Read the model definition and answer for the solid it produces. Units are mm, in the model's axes. Face numbers are marked on the shaded views. A direction names the side the tool comes from. Give positions to 0.01 mm unless a question says otherwise; leave off trailing zeros. Write each loop counter-clockwise with the first axis right and the second up, starting at its lowest first coordinate (ties: lowest second). Pieces come first, ordered by that corner, then holes. Notation, with made-up numbers: M 24.25,8.5 L 49.25,8.5 A18 ccw 49.25,38.5 Z; hole C 83,19.5 d11. An arc over 180 degrees is marked long. Write each question's results on one line, items separated by ' | '. Start each with the question number.
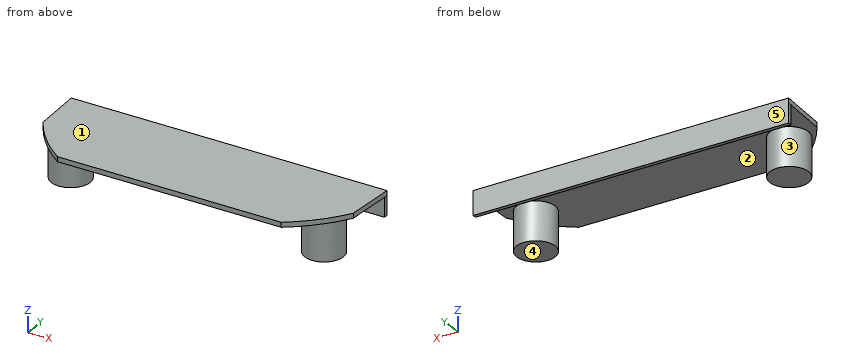
```python
from build123d import *

# Parameters (mm, degrees)
RESSALTO_EXTRUS_O1_DEPTH = 1.26
ESBO_O2_R                = 5
RESSALTO_EXTRUS_O2_DEPTH = 11.26
RESSALTO_EXTRUS_O3_DEPTH = 5


with BuildPart() as part:
    # Esboço1 → Ressalto-extrusão1 (new body)
    with BuildSketch(Plane.XY):
        with BuildLine():
            Line((0, 0), (58.25, 0))
            ThreePointArc((58.25, 0), (64.518594138, 5.422084196), (69.535183289, 12.019667297))
            Line((69.535183289, 12.019667297), (70.25, 25))
            Line((70.25, 25), (-12, 25))
            Line((-12, 25), (-11.285183289, 12.019667297))
            ThreePointArc((-11.285183289, 12.019667297), (-6.268594138, 5.422084196), (0, 0))
        make_face()
    extrude(amount=RESSALTO_EXTRUS_O1_DEPTH)

    # Esboço2 → Ressalto-extrusão2 (add)
    with BuildSketch(Plane.XY.offset(1.26)):
        with Locations((-3.61, 11.3)):
            Circle(ESBO_O2_R)
        with Locations((62.39, 11.3)):
            Circle(ESBO_O2_R)
    extrude(amount=-RESSALTO_EXTRUS_O2_DEPTH)

    # Esboço3 → Ressalto-extrusão3 (add)
    with BuildSketch(Plane(origin=(0, 0, 0), x_dir=(-1, 0, 0), z_dir=(0, 0, -1))):
        Polygon((-70.25, 25), (12, 25), (11.944930787, 24), (-70.194930787, 24), align=None)
    extrude(amount=RESSALTO_EXTRUS_O3_DEPTH)


solid = part.part
```
Item 1: Section C-C, the plane z = -8.25 is taken. Determine the outline of the cut face in (x, y).
Item 2: For the marked faces 1 and 2, determine the directions among +Z, -Z, +X, -X, +Y, -Y from which every point of the face is accessible in a straight line to the end or side of a thin tool.
Item 3: Section D-D, the plane y = 15.5 is taken. Determine the outline of the cut face in (x, z).
Item 4: Section B-B, the plane x = 48 is taken. Determine the outline of the cut face in (y, z), then the cut area to 3 significant figures.
Item 5: Determine the mould class of the marked faces 3, 4 and 5 for opening direction Y: +Y half, -Y half, draft (parallel to the pull), parting line (faces both ways), or undercut.
Item 6: Straight lines are drawn through the part: line 1 (X direction, y = 11.5, z = -3); line 2 (Y direction, x = 39, z = -4); line 3 (Z direction, x = 52.5, y = 3.5). For each, find the intervals that lie inside material, in ascending order.
Item 7: Section A-A, the plane z = -2.25 is taken. Determine the outline of the cut face in (x, y).
Item 8: Given P1, Ø5.5, axis at x = 14.5, z = -3, coming from the -Y side; P2, Ø7, axis at x = 29, y = 7.5, coming from the -Z side; P3, Ø10, axis at x = 42, y = 20, coming from the -Z side, each flat-ended and moving along its own axis, determine where each tip first touches the part or whether it passes through.
Worked out:
1) outline: C -3.61,11.3 d10; C 62.39,11.3 d10
2) face 1: +Z, +X, -X, +Y, -Y | face 2: -Z
3) outline: M -11.48,0 L -6.32,0 L -6.32,-10 L -0.9,-10 L -0.9,0 L 59.68,0 L 59.68,-10 L 65.1,-10 L 65.1,0 L 69.73,0 L 69.73,1.26 L -11.48,1.26 Z
4) outline: M 0,0 L 24,0 L 24,-5 L 25,-5 L 25,1.26 L 0,1.26 Z | area: 36.5 mm²
5) face 3: undercut | face 4: draft | face 5: +Y half
6) line 1: x = -8.61 to 1.39, 57.39 to 67.39 | line 2: y = 24 to 25 | line 3: z = 0 to 1.26
7) outline: M -12,25 L -11.94,24 L 70.19,24 L 70.25,25 Z; C -3.61,11.3 d10; C 62.39,11.3 d10
8) P1: stops at y = 24 | P2: stops at z = 0 | P3: stops at z = -5
